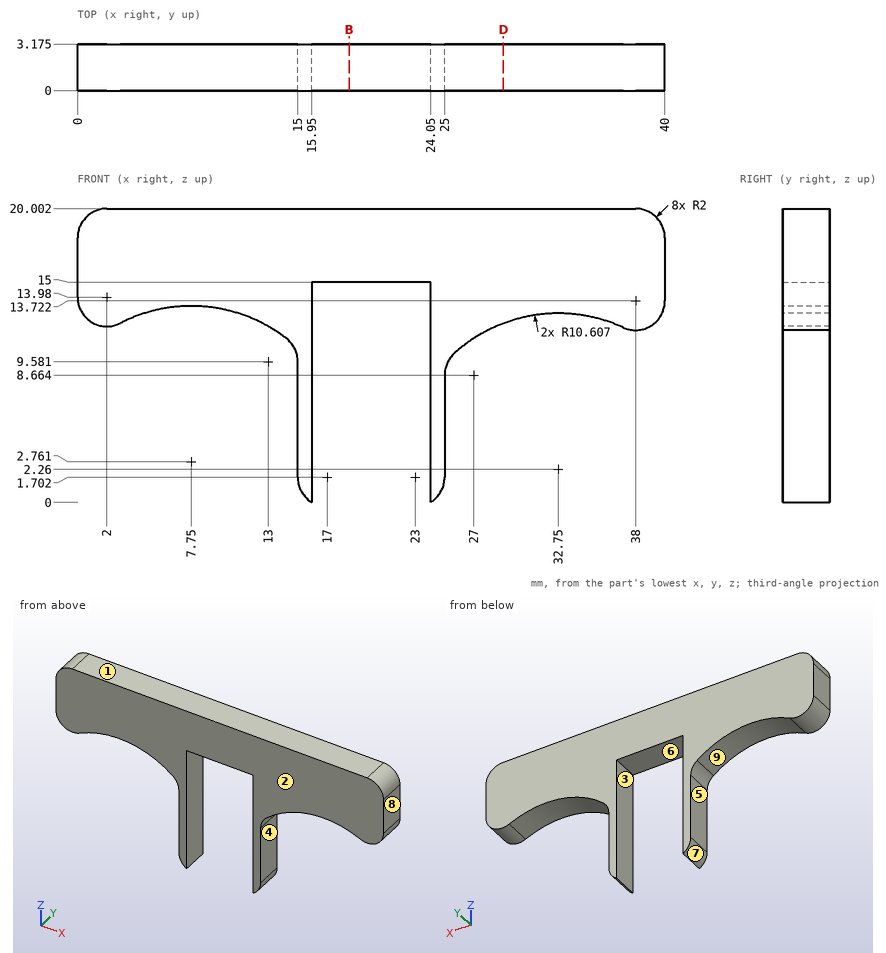
Job drawing, mm, ordinate dimensions from the low corner. One solid piece. A direction names the side the tool comes from. Round coordinates to 2 decimals unless told otherwise and drop trailing zeros. Write each loop counter-clockwise with the first axis right and the second up, starting at its lowest first coordinate (ties: lowest second). Pieces come first, ordered by that corner, then holes.
1) Pin check, flat tips, straight feed: pin 1 (1.5 mm diameter, centred on x = 32, y = 1, fed in from -Z); pin 2 (1 mm diameter, centred on y = 1.5, z = 6, fed in from +X); pin 3 (1 mm diameter, centred on y = 1, z = 11, fed in from -X). Stop position of each tip, or through.
2) Drill centre lines: probe 1 along X at (y, z) = (1.75, 7.25); probe 2 along X at (y, z) = (2.8, 14.25); probe 3 along Z at (x, y) = (19, 2.15). Where is each one in solid material? Low to high.
3) Mould opens along X. For the marked faces 6, 7, 8 and 9 say: +X half, -X half, draft (parallel to the pull), parting line (faces both ways), or undercut.
4) 3-axis set-ups, long thin cutter, end or side, ignore diameter. For the marked faces 1, 2, 3, 4 and 5: which of +Z, -Z, +X, -X, +Y, -Y reach the whole face in a straight line?
5) Band-saw the part on B-B, the plane x = 18.5. List the corners of the cut face in (y, z) (1 decimal), and give its area (3 significant figures).
6) Band-saw the part on D-D, the plane x = 29. List the corners of the cut face in (y, z) (1 decimal), and give its area (3 significant figures).
Ans:
1. pin 1: stops at z = 12.76
1. pin 2: stops at x = 25
1. pin 3: stops at x = 13.76
2. probe 1: x = 15 to 15.95, 24.05 to 25
2. probe 2: x = 0 to 15.95, 24.05 to 40
2. probe 3: z = 15 to 20
3. face 6: undercut
3. face 7: -X half
3. face 8: +X half
3. face 9: undercut
4. face 1: +Z, +X, -X, +Y, -Y
4. face 2: +Z, -Z, +X, -X, -Y
4. face 3: -Z, +Y, -Y
4. face 4: -Z, +X, +Y, -Y
4. face 5: -Z, -X, +Y, -Y
5. outline: (0, 15) - (3.2, 15) - (3.2, 20) - (0, 20) - close
5. area: 15.9 mm2
6. outline: (0, 12.2) - (3.2, 12.2) - (3.2, 20) - (0, 20) - close
6. area: 24.8 mm2
